Autodesk Inventor part; units mm, degrees
ref_plane "YZ Plane" through (0, 0, 0) normal (1, 0, 0) x (0, 1, 0)
ref_plane "XZ Plane" through (0, 0, 0) normal (0, 1, 0) x (-1, 0, 0)
ref_plane "XY Plane" through (0, 0, 0) normal (0, 0, 1) x (1, 0, 0)
sketch "スケッチ1" plane through (0, 0, 0) normal (0, 0, 1) x (1, 0, 0)
  line L0 (-63.6765, 0) -> (66.53, 0) construction
  line L1 (0, 73.5962) -> (0, -63.7716) construction
  circle A0 centre (0, 0) radius 5.05
  circle A1 centre (0, 0) radius 8 construction
  circle A2 centre (0, 0) radius 10.9
  circle A3 centre (0, 8.5) radius 1.35
  circle A4 centre (0, 8.5) radius 2.4 construction
  circle A5 centre (-8.5, 0) radius 2.4 construction
  circle A6 centre (-8.5, 0) radius 1.35
  circle A7 centre (0, -8.5) radius 2.4 construction
  circle A8 centre (0, -8.5) radius 1.35
  circle A9 centre (8.5, 0) radius 2.4 construction
  circle A10 centre (8.5, 0) radius 1.35
  line L2 (12.5, -41) -> (-12.5, -41)
  line L3 (-12.5, -41) -> (-12.5, -36)
  line L4 (-12.5, -36) -> (12.5, -36) construction
  line L5 (12.5, -36) -> (12.5, -41)
  line L6 (12.5, -41) -> (-12.5, -36) construction
  line L7 (-12.5, -41) -> (12.5, -36) construction
  line L8 (12.5, -36) -> (10.8894, 0.4808)
  line L9 (-12.5, -36) -> (-10.8894, 0.4808)
  circle A11 centre (-9.5, -38) radius 1.55
  line L10 (-12.5, -38) -> (12.5, -38) construction
  line L11 (-4.75, -36) -> (-4.75, -41) construction
  line L12 (4.75, -36) -> (4.75, -41) construction
  circle A12 centre (9.5, -38) radius 1.55
  line L13 (-4.75, -36) -> (4.75, -36) construction
  line L14 (4.75, -36) -> (4.75, -38.5) construction
  line L15 (4.75, -38.5) -> (-4.75, -38.5) construction
  line L16 (-4.75, -38.5) -> (-4.75, -36) construction
  line L17 (-4.75, -37.25) -> (4.75, -37.25) construction
  line L18 (-4.76, -38.51) -> (4.76, -38.51)
  line L19 (4.76, -38.51) -> (4.76, -35.99)
  line L20 (4.76, -35.99) -> (-4.76, -35.99)
  line L21 (-4.76, -35.99) -> (-4.76, -38.51)
  circle A13 centre (-3.71, -35.99) radius 1.05
  circle A14 centre (-3.71, -38.51) radius 1.05
  circle A15 centre (3.71, -35.99) radius 1.05
  circle A16 centre (3.71, -38.51) radius 1.05
  point P0 (0, -38.5)
  point P1 (4.75, -36)
  point P2 (2.66, -38.51)
  point P3 (-2.66, -38.51)
  point P4 (-2.66, -35.99)
  point P5 (2.66, -35.99)
  dimension "d0" = 10.1
  dimension "d1" = 16
  dimension "d4" = 2.7
  dimension "d5" = 8.5
  dimension "d6" = 4.8
  dimension "d10" = 360
  dimension "d12" = 25
  dimension "d13" = 5
  dimension "d14" = 36
  dimension "d15" = 3
  dimension "d16" = 9.5
  dimension "d17" = 3.1
  dimension "d18" = 3
  dimension "d19" = 4.75
  dimension "d30" = 19
  dimension "d39" = 0.01
  dimension "d40" = 1.05
  dimension "d41" = 2.1
extrude "押し出し1" add sketch "スケッチ1" along normal blind 2
equation "\"d19\" = 0.5 * d16"
properties part number "Foot_back_frame" material "アルミニウム 2014-T4"
Verification items for the finished model (mm, model axes). A direction names the side the tool comes from. Coordinates: 2 decimals unless noted, no trailing zeros. Write each loop counter-clockwise with the first axis right and the second up, starting at its lowest first coordinate (ties: lowest second). Pieces come first, ordered by that corner, then holes. Notation, with made-up numbers: M -40,77.25 L 12,77.25 A25 ccw 12,114.25 Z; hole C 6.5,7.5 d9. An arc over 180 degrees is marked long. Use a Markdown table: item, result.
Q1. Thickness scan on line 1 (Y direction, x = 0, z = 1.1); line 2 (Y direction, x = -4, z = 0.5); line 3 (Y direction, x = -3.5, z = 1.55). Record the ranges inside material, lowest first.
Reply:
| item | result |
|---|---|
| line 1 | y = -41 to -38.51, -35.99 to -9.85, -7.15 to -5.05, 5.05 to 7.15, 9.85 to 10.9 |
| line 2 | y = -41 to -39.52, -34.98 to -3.08, 3.08 to 10.14 |
| line 3 | y = -41 to -39.54, -34.96 to -3.64, 3.64 to 10.32 |
Q2. Sectioned sample at C-C, the plane z = 0.45. Count the separate pieces of the cut face and the enclosed holes in it, plus the area to 3 significant figures.
Reply:
| item | result |
|---|---|
| separate pieces | 1 |
| enclosed holes | 8 |
| area | 1,010 mm² |
Q3. Draft check along X on faces 1 (the face through (-12.5, -39, 1)), 2 (the face through (-0.2, 10.9, 1)), 3 (the face through (-7.212, -0.406, 0.986)), 4 (the face through (-9.836, -36.487, 0.986)). Enter one of: +X half, -X half, draft (parallel to the pull), parting line (faces both ways), or undercut.
Reply:
| item | result |
|---|---|
| face 1 | -X half |
| face 2 | parting line |
| face 3 | undercut |
| face 4 | undercut |
Q4. Sectioned sample at B-B, the plane y = -8.5. Record the boundary of the cut face in (x, z).
Reply:
| item | result |
|---|---|
| outline | M -11.29,0 L -1.35,0 L -1.35,2 L -11.29,2 Z; M 1.35,0 L 11.29,0 L 11.29,2 L 1.35,2 Z |
Q5. Go/stop test with a flat-tipped pin: P1, Ø2, axis at x = 0, y = -8.5, coming from the -Z side. Record where the tip stops, or that it passes through.
Reply:
| item | result |
|---|---|
| P1 | passes through |
Q6. Sectioned sample at A-A, the plane x = 0. Record the boundary of the cut face in (y, z), plus the area to 3 significant figures.
Reply:
| item | result |
|---|---|
| outline | M -41,0 L -38.51,0 L -38.51,2 L -41,2 Z; M -35.99,0 L -9.85,0 L -9.85,2 L -35.99,2 Z; M -7.15,0 L -5.05,0 L -5.05,2 L -7.15,2 Z; M 5.05,0 L 7.15,0 L 7.15,2 L 5.05,2 Z; M 9.85,0 L 10.9,0 L 10.9,2 L 9.85,2 Z |
| area | 67.8 mm² |
Q7. Sectioned sample at D-D, the plane x = 8.5. Record the boundary of the cut face in (y, z), plus the area to 3 significant figures.
Reply:
| item | result |
|---|---|
| outline | M -41,0 L -39.18,0 L -39.18,2 L -41,2 Z; M -36.82,0 L -1.35,0 L -1.35,2 L -36.82,2 Z; M 1.35,0 L 6.82,0 L 6.82,2 L 1.35,2 Z |
| area | 85.5 mm² |
Q8. Set-up check for faces 5 (the face through (0, -15, 2)), 6 (the face through (-3.69, -39.56, 0.99)): record each of +Z, -Z, +X, -X, +Y, -Y from which the full face is reachable in a straight line by a thin tool's end or side.
Reply:
| item | result |
|---|---|
| face 5 | +Z, +X, -X, +Y, -Y |
| face 6 | +Z, -Z |
